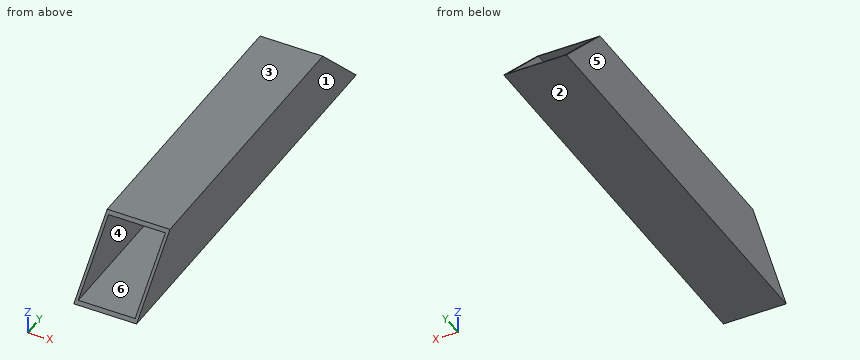
from build123d import *

# Parameters (mm, degrees)
SKETCH1_W           = 25.4
SKETCH1_H           = 25.4
SKETCH1_W_2         = 23
SKETCH1_H_2         = 23
BOSS_EXTRUDE1_DEPTH = 166.94
CUT_EXTRUDE1_DEPTH  = 26.4


with BuildPart() as part:
    # Sketch1 → Boss-Extrude1 (new body)
    with BuildSketch(Plane(origin=(0, 0, 0), x_dir=(1, 0, 0), z_dir=(0, 1, 0))):
        with Locations((12.7, 12.7)):
            Rectangle(SKETCH1_W, SKETCH1_H)
        with Locations((12.7, 12.7)):
            Rectangle(SKETCH1_W_2, SKETCH1_H_2, mode=Mode.SUBTRACT)
    extrude(amount=BOSS_EXTRUDE1_DEPTH)

    # Sketch2 → Cut-Extrude1 (cut, through all)
    with BuildSketch(Plane(origin=(25.4, 0, 0), x_dir=(0, 0, -1), z_dir=(1, 0, 0))):
        Polygon((25.4, 166.94), (0, 166.94), (0, 141.54), align=None)
        Polygon((0, 0), (0, 25.4), (25.4, 0), align=None)
    extrude(amount=-CUT_EXTRUDE1_DEPTH, mode=Mode.SUBTRACT)


solid = part.part
Design review of the part built by this model. Coordinates are the model's own, in mm. Face numbers are marked on the shaded views. A direction names the side the tool comes from. Round coordinates to 2 decimals unless told otherwise and drop trailing zeros. Write each loop counter-clockwise with the first axis right and the second up, starting at its lowest first coordinate (ties: lowest second). Pieces come first, ordered by that corner, then holes. Notation, with made-up numbers: (62.5, 1) -> (68.5, 1) arc R7 ccw to (68.5, 11) -> close; hole circle Ø10 at (19.5, 30). An arc over 180 degrees is marked (long way). One line per question, with ' | ' between items.
(1) Insertion check: P1, Ø8, axis at x = 14, z = -19.5, coming from the +Y side. The pin has a flat end and moves straight along its axis. Give the tip position at first contact, or say it passes through.
Result sheet:
P1: through
(2) Draft analysis for pull direction Z (two halves, no side actions). For the marked faces 1, 2, 3 and 4, state which applies: released by +Z, released by -Z, zero draft, split by the parting line, or undercut.
Result sheet:
face 1: zero draft | face 2: released by -Z | face 3: released by +Z | face 4: undercut
(3) Wall thickness on line 1 (X direction, y = 49, z = -8.5); line 2 (Z direction, x = 9.5, y = 107); line 3 (Z direction, x = 2.75, y = 21.5): over which ranges is each line inside the solid? List them lowest first. Write a range as [from, to].
Result sheet:
line 1: [0, 1.2], [24.2, 25.4] | line 2: [-25.4, -24.2], [-1.2, 0] | line 3: [-25.4, -24.2]
(4) Take a section at B-B, the plane x = 6.25. State the section outline as (y, z) points, and give its area (3 significant figures).
Result sheet:
outline: (0, -25.4) -> (166.94, -25.4) -> (165.74, -24.2) -> (1.2, -24.2) -> close; (24.2, -1.2) -> (142.74, -1.2) -> (141.54, 0) -> (25.4, 0) -> close | area: 340 mm2
(5) Machinability: for the marked faces 5 and 6, which of the approach directions +Z, -Z, +X, -X, +Y, -Y give a long, thin tool a straight path to every point of the face, cutting with its end or side? Answer none if there is none.
Result sheet:
face 5: +Z, -Z, -X, +Y, -Y | face 6: +Y, -Y
(6) Take a section at A-A, the plane z = -20.75. State the section outline as (x, y) points.
Result sheet:
outline: (0, 4.65) -> (1.2, 4.65) -> (1.2, 162.29) -> (0, 162.29) -> close; (24.2, 4.65) -> (25.4, 4.65) -> (25.4, 162.29) -> (24.2, 162.29) -> close
(7) Take a section at C-C, the plane y = 135. State the section outline as (x, z) points.
Result sheet:
outline: (0, -25.4) -> (25.4, -25.4) -> (25.4, 0) -> (0, 0) -> close; hole (1.2, -24.2) -> (24.2, -24.2) -> (24.2, -1.2) -> (1.2, -1.2) -> close
(8) Take a section at D-D, the plane y = 156. State the section outline as (x, z) points.
Result sheet:
outline: (0, -25.4) -> (25.4, -25.4) -> (25.4, -14.46) -> (24.2, -14.46) -> (24.2, -24.2) -> (1.2, -24.2) -> (1.2, -14.46) -> (0, -14.46) -> close
